Check sheet for the modelled part. Datum: model origin and axes. Units: mm. A direction names the side the tool comes from. Coordinates: 2 decimals unless noted, no trailing zeros. Loops run counter-clockwise (first coordinate to the right, second up) from the corner with the lowest first, then second, coordinate; pieces in that order, holes last.
Autodesk Inventor part; units mm, degrees
ref_plane "YZ Plane" through (0, 0, 0) normal (1, 0, 0) x (0, 1, 0)
ref_plane "XZ Plane" through (0, 0, 0) normal (0, 1, 0) x (-1, 0, 0)
ref_plane "XY Plane" through (0, 0, 0) normal (0, 0, 1) x (1, 0, 0)
sketch "Sketch1" plane through (0, 0, 0) normal (0, 0, 1) x (1, 0, 0)
  circle A0 centre (0, 0) radius 10.5
  circle A1 centre (0, 0) radius 4.5
  circle A2 centre (0, 0) radius 3
  line L0 (-15, 0) -> (15, 0) construction
  line L1 (0, -19) -> (0, 21.6238) construction
  circle A3 centre (0, -7.5) radius 0.5
  circle A4 centre (0, 7.5) radius 0.5
  circle A5 centre (0, 0) radius 1
  circle A6 centre (0, 0) radius 2.5
  dimension "d0" = 21
  dimension "d1" = 9
  dimension "d2" = 6
  dimension "d3" = 1
  dimension "d4" = 7.5
  dimension "d5" = 2
  dimension "d6" = 5
extrude "Extrusion1" add sketch "Sketch1" along normal blind 6 contours A1
extrude "Extrusion2" add sketch "Sketch1" along normal blind 2 contours A0 | A2 | A6
extrude "Extrusion3" cut sketch "Sketch1" along normal blind 1 contours A1 | A6
chamfer "Chamfer1" distance 0.5 angle 45 1 edges at (-4.5, 0, 6)
properties part number "ServoHorn"
1) Mould release check, pull along X, two halves, no side actions. Record for faces 4 (the flat face through (0, -5, 2)), 5 (the cylindrical face through (0, -7, 1)), 6 (the cylindrical face through (10, -3.2, 1)): +X half, -X half, draft (parallel to the pull), parting line (faces both ways), or undercut.
Answer sheet:
face 4: draft
face 5: undercut
face 6: parting line
2) Depth check by flat-ended pin: pin 1 (5 mm diameter, centred on x = -6.5, y = 4.5, fed in from +Z); pin 2 (4 mm diameter, centred on x = 0, y = 0, fed in from -Z); pin 3 (10 mm diameter, centred on x = -4, y = 4, fed in from +Z). Enter the tip coordinate at first touch or a pass-through.
Answer sheet:
pin 1: stops at z = 2
pin 2: stops at z = 1
pin 3: stops at z = 6
3) Section check C-C on x = 0. Give the number of separate pieces and of enclosed holes in the cut face, plus the area to 4 significant figures.
Answer sheet:
separate pieces: 4
enclosed holes: 0
area: 39.75 mm2
4) Set-up check for faces 1 (the cylindrical face through (-3, -0.1, 0.5)), 2 (the flat face through (0, -5, 0)), 3 (the cylindrical face through (-3, 0, 4)): record each of +Z, -Z, +X, -X, +Y, -Y from which the full face is reachable in a straight line by a thin tool's end or side.
Answer sheet:
face 1: -Z
face 2: -Z, +X, -X, +Y, -Y
face 3: +Z
5) Section check D-D on z = 2.7. Enter the section's corners in (x, y).
Answer sheet:
outline: circle Ø9 at (0, 0); hole circle Ø6 at (0, 0)
6) Scan lines: line 1 (Y direction, x = 0, z = 0.4); line 2 (Y direction, x = 0, z = 4.5); line 3 (Z direction, x = 0, y = 4.75). Record each from-to range of solid material in increasing order.
Answer sheet:
line 1: y = -10.5 to -8, -7 to -4.5, -3 to -2.5, 2.5 to 3, 4.5 to 7, 8 to 10.5
line 2: y = -4.5 to -3, 3 to 4.5
line 3: z = 0 to 2
7) Section check B-B on z = 0.7. Enter the section's corners in (x, y), plus the area to 3 significant figures.
Answer sheet:
outline: circle Ø21 at (0, 0); circle Ø6 at (0, 0); hole circle Ø9 at (0, 0); hole circle Ø5 at (0, 0); hole circle Ø1 at (0, -7.5); hole circle Ø1 at (0, 7.5)
area: 290 mm2
